from build123d import *

# Parameters (mm, degrees)
SKETCH1_W       = 60
SKETCH1_H       = 40
EXTRUDE1_DEPTH  = 70
EXTRUDE2_DEPTH  = 173.409396496
SKETCH5_R       = 7.5
EXTRUDE3_DEPTH  = 173.409396496
SKETCH8_R       = 11
EXTRUDE5_DEPTH  = 11
SKETCH9_W       = 15
SKETCH9_H       = 16.95
EXTRUDE6_DEPTH  = 173.409396496
SKETCH10_W      = 22
SKETCH10_H      = 31.344818361
EXTRUDE7_DEPTH  = 11
SKETCH13_W      = 3
SKETCH13_H      = 17
EXTRUDE9_DEPTH  = 3
SKETCH14_W      = 3
SKETCH14_H      = 17
EXTRUDE10_DEPTH = 3
SKETCH16_W      = 3
SKETCH16_H      = 37
EXTRUDE11_DEPTH = 41
SKETCH17_W      = 3
SKETCH17_H      = 37
EXTRUDE12_DEPTH = 6
SKETCH18_W      = 3
SKETCH18_H      = 10
EXTRUDE13_DEPTH = 33
SKETCH19_W      = 3
SKETCH19_H      = 3
EXTRUDE14_DEPTH = 10
FILLET1_R       = 3
SKETCH20_R      = 2
EXTRUDE15_DEPTH = 5
FILLET2_R       = 2
FILLET3_R       = 2
EXTRUDE16_DEPTH = 40
FILLET4_RADIUS  = 20
FILLET4_LENGTH  = 2.6
EXTRUDE17_DEPTH = 2.6
SKETCH24_R      = 1
EXTRUDE18_DEPTH = 2.6
SKETCH25_R      = 2.5
EXTRUDE19_DEPTH = 2.6
SKETCH26_R      = 6
EXTRUDE20_DEPTH = 5
SKETCH27_R      = 6
EXTRUDE21_DEPTH = 2.6
SKETCH28_R      = 7
EXTRUDE22_DEPTH = 1
SKETCH29_R      = 19.5
EXTRUDE23_DEPTH = 18
SKETCH30_R      = 15
EXTRUDE24_DEPTH = 28
SKETCH31_W      = 1.052605107
SKETCH31_H      = 2.780967683
SKETCH31_W_2    = 1.226574425
EXTRUDE25_DEPTH = 3


with BuildPart() as part:
    # Sketch1 → Extrude1 (new body)
    with BuildSketch(Plane(origin=(0, 5, 0), x_dir=(1, 0, 0), z_dir=(0, 1, 0))):
        with Locations((-120, 0)):
            Rectangle(SKETCH1_W, SKETCH1_H)
    extrude(amount=EXTRUDE1_DEPTH)

    # Sketch4 → Extrude2 (cut, through all)
    with BuildSketch(Plane.XY.offset(20)):
        Polygon((-106.8, 75), (-106.8, 38), (-69.340811885, 38), (-69.340811885, 101.678315396), (-106.8, 101.678315396), align=None)
    extrude(amount=-EXTRUDE2_DEPTH, mode=Mode.SUBTRACT)

    # Sketch5 → Extrude3 (cut, through all)
    with BuildSketch(Plane.XY.offset(20)):
        with Locations((-120, 58.05)):
            Circle(SKETCH5_R)
    extrude(amount=-EXTRUDE3_DEPTH, mode=Mode.SUBTRACT)

    # Sketch8 → Extrude5 (cut, symmetric)
    with BuildSketch(Plane.XY):
        with Locations((-120, 58.05)):
            Circle(SKETCH8_R)
    extrude(amount=EXTRUDE5_DEPTH, both=True, mode=Mode.SUBTRACT)

    # Sketch9 → Extrude6 (cut, through all)
    with BuildSketch(Plane.XY.offset(20)):
        with Locations((-120, 66.525)):
            Rectangle(SKETCH9_W, SKETCH9_H)
    extrude(amount=-EXTRUDE6_DEPTH, mode=Mode.SUBTRACT)

    # Sketch10 → Extrude7 (cut, symmetric)
    with BuildSketch(Plane.XY):
        with Locations((-120, 73.722409181)):
            Rectangle(SKETCH10_W, SKETCH10_H)
    extrude(amount=EXTRUDE7_DEPTH, both=True, mode=Mode.SUBTRACT)

    # Sketch13 → Extrude9 (cut)
    with BuildSketch(Plane(origin=(-127.5, 0, 0), x_dir=(0, 0, -1), z_dir=(1, 0, 0))):
        with Locations((-15.5, 66.5)):
            Rectangle(SKETCH13_W, SKETCH13_H)
    extrude9 = extrude(amount=-EXTRUDE9_DEPTH, mode=Mode.SUBTRACT)

    # Sketch14 → Extrude10 (cut)
    with BuildSketch(Plane.ZY.offset(112.5)):
        with Locations((15.5, 66.5)):
            Rectangle(SKETCH14_W, SKETCH14_H)
    extrude10 = extrude(amount=-EXTRUDE10_DEPTH, mode=Mode.SUBTRACT)

    # Mirror1: Extrude9, Extrude10 across plane
    add(extrude9.mirror(Plane.XY), mode=Mode.SUBTRACT)
    add(extrude10.mirror(Plane.XY), mode=Mode.SUBTRACT)

    # Sketch16 → Extrude11 (add)
    with BuildSketch(Plane.XY.offset(-17)):
        with Locations((-102.3, 56.5)):
            Rectangle(SKETCH16_W, SKETCH16_H)
    extrude(amount=EXTRUDE11_DEPTH)

    # Sketch17 → Extrude12 (add)
    with BuildSketch(Plane(origin=(-100.8, 0, 0), x_dir=(0, 0, -1), z_dir=(1, 0, 0))):
        with Locations((18.5, 56.5)):
            Rectangle(SKETCH17_W, SKETCH17_H)
    extrude(amount=-EXTRUDE12_DEPTH)

    # Sketch18 → Extrude13 (add)
    with BuildSketch(Plane.XZ.offset(-38)):
        with Locations((-102.3, 25)):
            Rectangle(SKETCH18_W, SKETCH18_H)
    extrude(amount=EXTRUDE13_DEPTH)

    # Sketch19 → Extrude14 (add)
    with BuildSketch(Plane(origin=(0, 38, 0), x_dir=(1, 0, 0), z_dir=(0, 1, 0))):
        with Locations((-102.3, -28.5)):
            Rectangle(SKETCH19_W, SKETCH19_H)
    extrude(amount=EXTRUDE14_DEPTH)

    # Fillet1
    fillet1_edges = [part.edges().sort_by_distance(p)[0] for p in [
        (-100.8, 38, 0),
        (-100.8, 21.5, 20),
        (-103.8, 21.5, 20),
    ]]
    fillet(fillet1_edges, radius=FILLET1_R)

    # Sketch20 → Extrude15 (add)
    with BuildSketch(Plane.XZ.offset(-5)):
        with BuildLine():
            Line((-156, 4), (-150, 4))
            Line((-150, 4), (-150, -4))
            Line((-150, -4), (-156, -4))
            ThreePointArc((-156, -4), (-160, 0), (-156, 4))
        make_face()
        with Locations(Location((-156, 0, 0), (0, 0, 270))):
            Circle(SKETCH20_R, mode=Mode.SUBTRACT)
    extrude15 = extrude(amount=-EXTRUDE15_DEPTH)

    # Fillet2
    fillet2_edges = [part.edges().sort_by_distance(p)[0] for p in [
        (-150, 10, 0),
        (-150, 7.5, 4),
        (-150, 7.5, -4),
    ]]
    fillet(fillet2_edges, radius=FILLET2_R)

    # Mirror7: Extrude15 across plane
    add(extrude15.mirror(Plane.ZY.offset(120)))

    # Fillet3
    fillet3_edges = [part.edges().sort_by_distance(p)[0] for p in [
        (-90, 10, 0),
        (-90, 7.5, -4),
        (-90, 7.5, 4),
    ]]
    fillet(fillet3_edges, radius=FILLET3_R)

    # Sketch21 → Extrude16 (add)
    with BuildSketch(Plane(origin=(0, 38, 0), x_dir=(1, 0, 0), z_dir=(0, 1, 0))):
        Polygon((-104, -21.450806662), (-104, 16.8), (-106.6, 16.8), (-106.6, -19.806256115), (-106.6, -26.8), (-103.6, -26.8), (-101, -26.8), (-60.6, -26.8), (-60.6, -24.2), (-101, -24.2), (-103.6, -24.2), (-104, -24.2), align=None)
    extrude(amount=EXTRUDE16_DEPTH)

    # Fillet4: full round fillet: the end face becomes a half cylinder, R = half its width
    fillet4_face = Plane((-60.6, 58, 25.5), x_dir=(0, 0, -1), z_dir=(1, 0, 0))  # on the end face: x along it, z out of the body
    fillet4_slab = fillet4_face.offset(-FILLET4_RADIUS / 2) * Box(FILLET4_LENGTH, 2 * FILLET4_RADIUS, FILLET4_RADIUS, mode=Mode.PRIVATE)  # the body's end, R deep
    fillet4_round = Plane((-80.6, 58, 25.5), x_dir=(1, 0, 0), z_dir=(0, 0, -1)) * Cylinder(FILLET4_RADIUS, FILLET4_LENGTH, mode=Mode.PRIVATE)  # its axis R under the face
    add(fillet4_slab - fillet4_round, mode=Mode.SUBTRACT)

    # Sketch22 → Extrude17 (cut)
    with BuildSketch(Plane.XY.offset(26.8)):
        with BuildLine():
            Line((-89.6, 51.5), (-75.6, 51.5))
            ThreePointArc((-75.6, 51.5), (-69.1, 58), (-75.6, 64.5))
            Line((-75.6, 64.5), (-89.6, 64.5))
            ThreePointArc((-89.6, 64.5), (-96.1, 58), (-89.6, 51.5))
        make_face()
    extrude(amount=-EXTRUDE17_DEPTH, mode=Mode.SUBTRACT)

    # Sketch24 → Extrude18 (cut)
    with BuildSketch(Plane.XY.offset(26.8)):
        with Locations((-65.470800536, 58)):
            Circle(SKETCH24_R)
        with Locations((-74.138374008, 42.987322368)):
            Circle(SKETCH24_R)
        with Locations((-91.473520952, 42.987322368)):
            Circle(SKETCH24_R)
        with Locations((-100.141094423, 58)):
            Circle(SKETCH24_R)
        with Locations((-91.473520952, 73.012677632)):
            Circle(SKETCH24_R)
        with Locations((-74.138374008, 73.012677632)):
            Circle(SKETCH24_R)
    extrude(amount=-EXTRUDE18_DEPTH, mode=Mode.SUBTRACT)

    # Sketch25 → Extrude19 (add)
    with BuildSketch(Plane.XY.offset(26.8)):
        with Locations((-100.141094423, 58)):
            Circle(SKETCH25_R)
    extrude(amount=-EXTRUDE19_DEPTH)



with BuildPart() as body_2:
    # Sketch26 → Extrude20 (new body)
    with BuildSketch(Plane.XY.offset(26.8)):
        with Locations((-86, 58)):
            Circle(SKETCH26_R)
    extrude(amount=EXTRUDE20_DEPTH)

    # Sketch27 → Extrude21 (add)
    with BuildSketch(Plane(origin=(0, 0, 26.8), x_dir=(-1, 0, 0), z_dir=(0, 0, -1))):
        with Locations(Location((86, 58, 0), (0, 0, 180))):
            Circle(SKETCH27_R)
    extrude(amount=EXTRUDE21_DEPTH)


with BuildPart() as part_1:
    add(part.part)

    add(body_2.part)  # Extrude22 merges body 2
    # Sketch28 → Extrude22 (add)
    with BuildSketch(Plane(origin=(0, 0, 24.2), x_dir=(-1, 0, 0), z_dir=(0, 0, -1))):
        with Locations(Location((86, 58, 0), (0, 0, 111.786789298))):
            Circle(SKETCH28_R)
    extrude(amount=EXTRUDE22_DEPTH)

    # Sketch29 → Extrude23 (add)
    with BuildSketch(Plane(origin=(0, 0, 23.2), x_dir=(-1, 0, 0), z_dir=(0, 0, -1))):
        with Locations((82.736652481, 57.95294162)):
            Circle(SKETCH29_R)
    extrude(amount=EXTRUDE23_DEPTH)

    # Sketch30 → Extrude24 (add)
    with BuildSketch(Plane(origin=(0, 0, 5.2), x_dir=(-1, 0, 0), z_dir=(0, 0, -1))):
        with Locations(Location((82.736652481, 57.95294162, 0), (0, 0, 180))):
            Circle(SKETCH30_R)
    extrude(amount=EXTRUDE24_DEPTH)

    # Sketch31 → Extrude25 (add)
    with BuildSketch(Plane(origin=(0, 0, -22.8), x_dir=(-1, 0, 0), z_dir=(0, 0, -1))):
        with Locations((70.766955126, 57.275867088)):
            Rectangle(SKETCH31_W, SKETCH31_H)
        with Locations((95.278427538, 57.275867088)):
            Rectangle(SKETCH31_W_2, SKETCH31_H)
    extrude(amount=EXTRUDE25_DEPTH)


solid = part_1.part
Check sheet for the modelled part. Datum: model origin and axes. Units: mm. A direction names the side the tool comes from. Round coordinates to 2 decimals unless told otherwise and drop trailing zeros. Loops run counter-clockwise (first coordinate to the right, second up) from the corner with the lowest first, then second, coordinate; pieces in that order, holes last. Notation, with made-up numbers: (45.25, 43) -> (61.25, 43) arc R12 cw to (61.25, 61) -> close; hole circle Ø8 at (-24, 29.25). An arc over 180 degrees is marked (long way). Put each result on its own line as item: value. Start each with the question number.
1. Section check C-C (x = -120). Enter the section's corners in (y, z), plus the area to 4 significant figures.
2. Scan lines: probe 1 along Z at (x, y) = (-110, 71.5); probe 2 along X at (y, z) = (69.5, -5); probe 3 along Z at (x, y) = (-156, 7.6). Record each from-to range of solid material in increasing order.
3. Access from +Z, -Z, +X, -X, +Y, -Y to the whole of each face (thin tool, end or side, straight path). Record for faces 5 (the face through (-130.5, 67, -16)), 6 (the face through (-86, 7, -4)), 7 (the face through (-127.5, 66, -12)).
4. Section check A-A (z = -7.5). Enter the section's corners in (x, y).
5. Gauge pin test, flat ends, axial feed: pin 1 (0.9 mm diameter, centred on x = -111.5, y = 65, fed in from -Z); pin 2 (2 mm diameter, centred on x = -79.5, z = 25, fed in from -Y); pin 3 (4 mm diameter, centred on y = 56.5, z = 14.5, fed in from -X); pin 4 (6.5 mm diameter, centred on x = -119.5, y = 55, fed in from +Z). Record the tip position at first contact, or that the pin passes through.
6. Section check B-B (y = 20). Enter the section's corners in (x, z).
7. Draft check along X on faces 1 (the face through (-94, 21, 20)), 2 (the face through (-70.241, 57, -24)), 3 (the face through (-120.16, 50.55, 15.56)), 4 (the face through (-160, 7, 0)). Enter one of: +X half, -X half, draft (parallel to the pull), parting line (faces both ways), or undercut.
8. Section check D-D (z = 0). Give the number of separate pieces and of enclosed holes in the cut face, plus the area to 3 significant figures.
Findings:
1. outline: (5, -20) -> (50.55, -20) -> (50.55, -11) -> (47.05, -11) -> (47.05, 11) -> (50.55, 11) -> (50.55, 20) -> (5, 20) -> close
1. area: 1,745 mm^2
2. probe 1: z = -20 to -17, -14 to -11, 11 to 14, 17 to 20
2. probe 2: x = -150 to -131, -109 to -106.8, -106.6 to -104, -103.8 to -100.8, -92.31 to -73.16
2. probe 3: z = -4 to -2, 2 to 4
3. face 5: +Y
3. face 6: -Z, +X, -Y
3. face 7: +Z, -Z, +Y
4. outline: (-150, 5) -> (-90, 5) -> (-90, 38) -> (-97.8, 38) arc R3 cw to (-100.8, 41) -> (-100.8, 75) -> (-103.8, 75) -> (-103.8, 38) -> (-104, 38) -> (-104, 78) -> (-106.6, 78) -> (-106.6, 38) -> (-106.8, 38) -> (-106.8, 75) -> (-109, 75) -> (-109, 58.05) arc R11 cw to (-131, 58.05) -> (-131, 75) -> (-150, 75) -> close; circle Ø30 at (-82.74, 57.95)
5. pin 1: stops at z = -20
5. pin 2: stops at y = 38
5. pin 3: stops at x = -150
5. pin 4: passes through
6. outline: (-150, -20) -> (-90, -20) -> (-90, 20) -> (-97.8, 20) arc R3 cw to (-100.8, 23) -> (-100.8, 30) -> (-103.8, 30) -> (-103.8, 23) arc R3 cw to (-106.8, 20) -> (-150, 20) -> close
7. face 1: draft
7. face 2: +X half
7. face 3: undercut
7. face 4: -X half
8. separate pieces: 4
8. enclosed holes: 0
8. area: 4,000 mm^2
